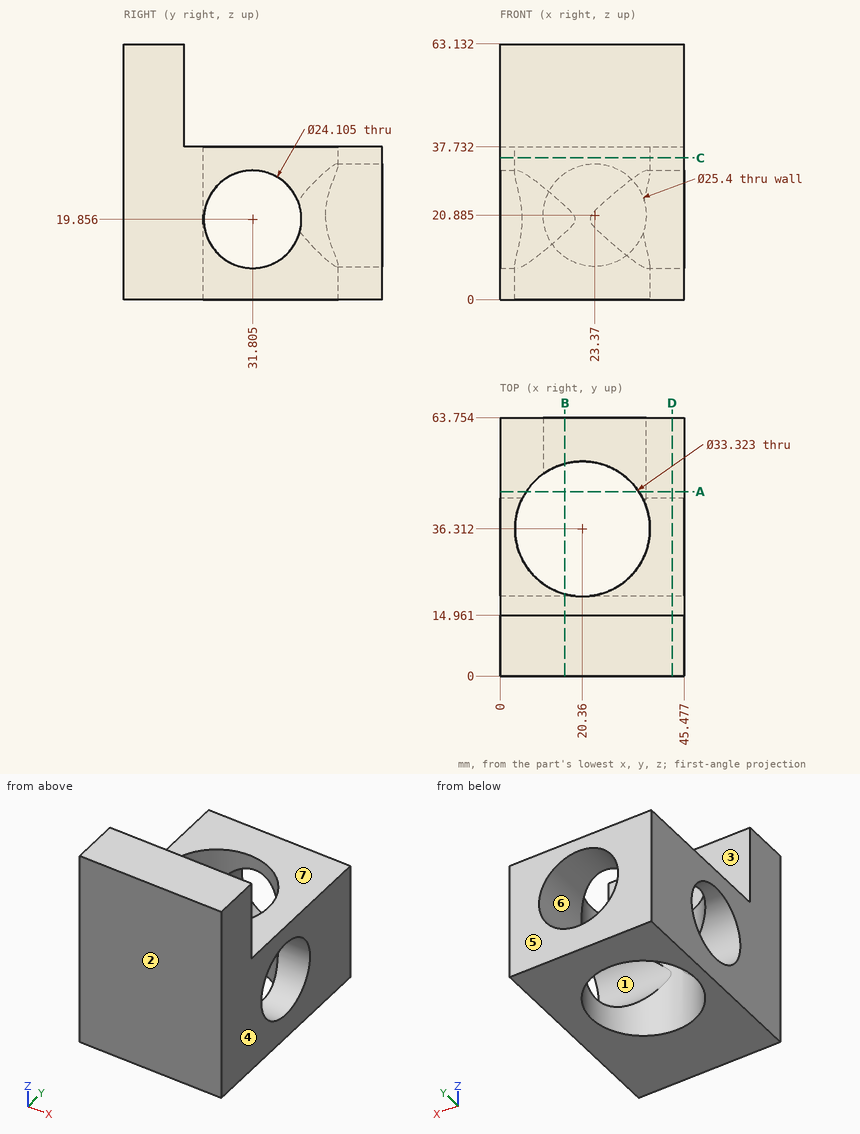
Geometry: see drawing. Coordinates: mm, zero at the bounding-box minimum. A direction names the side the tool comes from. Give positions to 0.01 mm unless a question says otherwise; leave off trailing zeros. Loops run counter-clockwise (first coordinate to the right, second up) from the corner with the lowest first, then second, coordinate; pieces in that order, holes last. Notation, with made-up numbers: (2, -36.5) -> (60, -36.5) arc R20 ccw to (60, -12.5) -> close; hole circle Ø9 at (81, -23.75). An arc over 180 degrees is marked (long way). Use one line per item in the form item = value.
Item 1: Section query D-D on x = 42.5. Output: boundary loops of the cut face in (y, z) (1 decimal).
A:
outline = (0, 0) -> (63.8, 0) -> (63.8, 37.7) -> (15, 37.7) -> (15, 63.1) -> (0, 63.1) -> close; hole circle Ø24.1 at (31.8, 19.9)
Item 2: Pin query (flat end, axial travel): P1, Ø10, axis at y = 51.5, z = 40.5, coming from the -X side; P2, Ø22.5, axis at x = 14, y = 35, coming from the +Z side; P3, Ø4, axis at x = 33, z = 51.5, coming from the +Y side. Return the tip coordinate at first contact, or that it passes through.
A:
P1 = 0
P2 = 37.73
P3 = 14.96
Item 3: Section query A-A on y = 45.5. Output: boundary loops of the cut face in (x, z) (1 decimal).
A:
outline = (0, 0) -> (6.5, 0) -> (6.5, 37.7) -> (0, 37.7) -> close; (34.3, 0) -> (45.5, 0) -> (45.5, 37.7) -> (34.3, 37.7) -> (34.3, 27.4) arc R12.7 cw to (34.3, 14.3) -> close
Item 4: Access query for the marked faces 5, 6 and 7. Directions: +Z, -Z, +X, -X, +Y, -Y. A direction counts if a zero-diameter tool reaches every point of the face in a straight line with its end or side. Return the directions, or none.
A:
face_5 = +Z, -Z, +X, -X, +Y
face_6 = +Y
face_7 = +Z, +X, -X, +Y
Item 5: Line query: probe 1 along Y at (x, z) = (3, 55.5); probe 2 along Y at (x, z) = (7.5, 37.5) (1 decimal); probe 3 along Y at (x, z) = (16.5, 36.5) (1 decimal). Output: solid intervals per line, ascending.
A:
probe_1 = 0 to 14.96
probe_2 = 0 to 25.7, 46.9 to 63.8
probe_3 = 0 to 20.1, 52.5 to 63.8
Item 6: Section query B-B on x = 16. Output: boundary loops of the cut face in (y, z) (1 decimal), and give its area (4 significant figures).
A:
outline = (0, 0) -> (20.2, 0) -> (20.2, 16.5) arc R12.1 cw to (20.2, 23.2) -> (20.2, 37.7) -> (15, 37.7) -> (15, 63.1) -> (0, 63.1) -> close; (52.4, 0) -> (63.8, 0) -> (63.8, 10.5) -> (52.4, 10.5) -> close; (52.4, 31.2) -> (63.8, 31.2) -> (63.8, 37.7) -> (52.4, 37.7) -> close
area = 1,335 mm^2
Item 7: Draft query along Y for the marked faces 1, 2, 3 and 4. Return one class per face: pulls with the +Y half, pulls with the -Y half, needs draft (parallel to the pull), parting line crosses it, or undercut.
A:
face_1 = undercut
face_2 = pulls with the -Y half
face_3 = pulls with the +Y half
face_4 = needs draft
Item 8: Section query C-C on z = 35. Output: boundary loops of the cut face in (x, y).
A:
outline = (0, 0) -> (45.48, 0) -> (45.48, 63.75) -> (0, 63.75) -> close; hole circle Ø33.32 at (20.36, 36.31)
